Autodesk Inventor part; units mm, degrees
ref_plane "YZ Plane" through (0, 0, 0) normal (1, 0, 0) x (0, 1, 0)
ref_plane "XZ Plane" through (0, 0, 0) normal (0, 1, 0) x (-1, 0, 0)
ref_plane "XY Plane" through (0, 0, 0) normal (0, 0, 1) x (1, 0, 0)
sketch "Sketch1" plane through (0, 0, 0) normal (0, 0, 1) x (1, 0, 0)
  line L0 (0, 6.1628) -> (0, 4.6128)
  line L1 (0, 0) -> (0, -5.3285)
  line L2 (0, -7.6236) -> (0, 6.1628)
  line L3 (7.7918, 0) -> (42.6907, 0)
  line L4 (6.1094, -12.088) -> (6.1094, -4.669)
  line L5 (-6.1094, -10.2236) -> (-6.1094, -4.5067)
  line L6 (0, -7.6236) -> (0, -10.2236)
  line L7 (0, -7.6236) -> (0, -5.0236) construction
  arc A0 (-6.1094, 5.0092) -> (-6.87, -3.5101) centre (0, 0.1701) ccw
  arc A1 (6.1094, -4.669) -> (4.9829, 6.1628) centre (0, 0.1701) ccw
  circle A2 centre (27.3823, 0) radius 1.6
  circle A3 centre (27.3823, 0) radius 1.6
  arc A4 (15.7262, -19.2861) -> (15.9651, 19.4308) centre (0.0053, 0.1701) ccw
  arc A5 (14.9776, -18.1086) -> (14.9776, 18.1086) centre (0, 0) ccw construction
  line L8 (25.0186, 0.0157) -> (19.4598, 0.0157) construction
  line L9 (22.9824, -8.2534) -> (24.1975, 0.0157) construction
  line L10 (24.1975, 0.0157) -> (22.8643, 8.3172) construction
  line L11 (28.9823, 0) -> (30.9823, 0) construction
  line L12 (33.1204, -3.5101) -> (30.9986, 0.1649)
  line L13 (39.4857, -3.5101) -> (33.1204, -3.5101)
  line L14 (39.4857, 0.1649) -> (37.3639, -3.5101)
  circle A6 centre (35.2258, 0) radius 1.9
  line L15 (30.9986, 0.1649) -> (33.1239, 3.846)
  line L16 (33.1239, 3.846) -> (39.4857, 3.8504)
  line L17 (37.3639, 3.8489) -> (39.4857, 0.1649)
  line L18 (39.4857, 0.1784) -> (39.4857, 3.8504)
  line L19 (39.4857, 3.8504) -> (39.4857, -3.5101)
  line L20 (39.4857, 3.8504) -> (39.4857, 5.8504)
  line L21 (39.4857, 5.8504) -> (23.6696, 8.2698)
  arc A7 (15.7262, -19.2861) -> (15.9651, 19.4308) centre (0, 0.1701) ccw
  line L22 (39.4857, -3.5101) -> (39.4857, -5.5101)
  line L23 (39.4857, -5.5101) -> (23.6696, -7.9296)
  line L24 (23.6696, -7.9296) -> (23.6696, 8.2698)
  line L25 (0, 6.1628) -> (0, -10.2236)
  line L26 (0, -12.323) -> (0, -15.7561)
  line L27 (10.9155, -5.0236) -> (17.2808, -5.0236)
  line L28 (17.2808, -8.6986) -> (15.159, -12.3736)
  circle A8 centre (13.0373, -8.6986) radius 1.9
  line L29 (8.7937, -8.6986) -> (10.9155, -5.0236)
  line L30 (17.2808, -12.3736) -> (10.9155, -12.3736)
  line L31 (10.9155, -12.3736) -> (8.7937, -8.6986)
  line L32 (15.159, -5.0236) -> (17.2808, -8.6986)
  line L33 (10.9155, -12.3736) -> (10.9155, -14.3736)
  line L34 (-6.1094, -10.2236) -> (-6.1094, -14.3736)
  line L35 (0, -14.3736) -> (0, -10.2236)
  line L36 (0, -14.3736) -> (0, -19.3736)
  line L37 (-6.1094, -19.3736) -> (-6.1094, -14.3736)
  line L38 (0, -19.3736) -> (0, -25.3736)
  line L39 (0, -25.3736) -> (-6.1094, -25.3736)
  line L40 (-6.1094, -25.3736) -> (-6.1094, -19.3736)
  arc A9 (-4.8255, 6.1628) -> (-6.1094, -4.5067) centre (0, 0.1701) ccw
  line L41 (-5.029, 6.1628) -> (-4.9829, 6.1628)
  line L42 (-4.8255, 6.1628) -> (0, 6.1628)
  dimension "d2" = 3.8
  dimension "d3" = 2
  dimension "d4" = 2
  dimension "d5" = 16
  dimension "d6" = 2
  dimension "d7" = 16
  dimension "d9" = 3.8
  dimension "d10" = 2
  dimension "d17" = 5
  dimension "d50" = 6
  dimension "d64" = 7.7937
  dimension "d65" = 15.388
revolve "Revolution1" add sketch "Sketch1" angle 360 about axis through (0, -12.323, 0) along (0, -1, 0) contours L0 L2 L1 L6 L35 L26 L36 L38 L39 L40 L37 L34 L5 A9 L42
sketch "Sketch2" plane through (0, 0, 0) normal (1, 0, 0) x (0, 1, 0)
  line L0 (-4.669, 0) -> (-6.7907, -3.675) construction
  line L1 (-6.7907, 3.675) -> (-4.669, 0) construction
  line L2 (-15.156, 0) -> (-13.156, 0) construction
  line L3 (-11.0343, -3.675) -> (-6.7907, -3.675) construction
  line L4 (-4.5067, -6.1094) -> (-4.5067, 6.1094) construction
  line L5 (-4.5067, -6.1094) -> (-4.5067, 6.1094) construction
  line L6 (-48.8073, 0) -> (-58.5119, 0) construction
  line L7 (-8.9125, 0) -> (-6.3144, -1.5) construction
  line L8 (-17.8945, -2.9836) -> (-21.3586, -2.9836)
  line L9 (-21.3586, -2.9836) -> (-23.0907, 0.0164)
  line L10 (-23.0907, 0.0164) -> (-21.3586, 3.0164)
  line L11 (-21.3586, 3.0164) -> (-17.8945, 3.0164)
  line L12 (-17.8945, 3.0164) -> (-16.1625, 0.0164)
  line L13 (-16.1625, 0.0164) -> (-17.8945, -2.9836)
  line L14 (23.6533, 6.6124) -> (23.3606, 8.9041) construction
  line L15 (29.9823, 11.5805) -> (34.9823, 11.5805) construction
  line L16 (24.1789, 0) -> (22.8458, 8.3015) construction
  line L17 (25, 0) -> (19.4412, 0) construction
  line L18 (25.1551, -0.0164) -> (29.5051, -0.0164) construction
  line L19 (23.6533, -6.0645) -> (23.6533, 6.6124) construction
  arc A0 (14.9776, -18.1086) -> (14.9776, 18.1086) centre (0, 0) ccw construction
  arc A1 (18.0021, -17.3472) -> (18.0021, 17.3472) centre (0, 0) ccw construction
  arc A2 (18.0021, -17.3472) -> (18.0021, 17.3472) centre (0, 0) ccw construction
  line L20 (22.9638, -8.2692) -> (24.1789, 0) construction
  circle A3 centre (29.5051, -0.0164) radius 4.35 construction
  line L21 (43.4694, -5.828) -> (23.3606, -8.9041) construction
  line L22 (43.4694, 5.828) -> (23.3606, 8.9041) construction
  line L23 (37.4871, -3) -> (35.7551, 0) construction
  line L24 (35.7551, 0) -> (37.4871, 3) construction
  line L25 (43.4694, 5.828) -> (43.4694, -5.828) construction
  circle A4 centre (39.2192, 0) radius 1.9 construction
  line L26 (25, 0) -> (20.4835, 0) construction
  line L27 (23.6533, -6.0645) -> (23.3606, -8.9041) construction
  line L28 (43.4694, 0) -> (43.4694, 5.828) construction
  line L29 (43.4694, -5.828) -> (43.4694, 5.828) construction
  line L30 (29.5346, 0.0703) -> (29.5346, 0.0867) construction
  line L31 (37.4871, 3) -> (43.4694, 3.5234) construction
  line L32 (37.4871, -3) -> (43.4694, -3.5234) construction
  circle A5 centre (-17.0481, 18.2856) radius 1.75
  line L33 (-15.4481, 18.2856) -> (-13.4481, 18.2856) construction
  line L34 (-11.3263, 14.6106) -> (-13.4481, 18.2856) construction
  line L35 (-13.4481, 18.2856) -> (-11.3263, 21.9606) construction
  circle A6 centre (-9.2045, 18.2856) radius 1.9
  line L36 (-4.961, 18.2856) -> (-7.0828, 14.6106) construction
  line L37 (-7.0828, 21.9606) -> (-4.961, 18.2856) construction
  line L38 (-11.3263, 21.9606) -> (-7.0828, 21.9606) construction
  line L39 (-11.3263, 14.6106) -> (-7.0828, 14.6106) construction
  line L40 (-9.2045, 18.2856) -> (-6.6065, 16.7856)
  line L41 (-7.4725, 15.2856) -> (-10.9366, 15.2856)
  line L42 (-10.9366, 15.2856) -> (-12.6686, 18.2856)
  line L43 (-12.6686, 18.2856) -> (-10.9366, 21.2856)
  line L44 (-10.9366, 21.2856) -> (-7.4725, 21.2856)
  line L45 (-7.4725, 21.2856) -> (-5.7404, 18.2856)
  line L46 (-5.7404, 18.2856) -> (-7.4725, 15.2856)
  circle A7 centre (-19.6266, 0.0164) radius 1.9 construction
  circle A8 centre (-9.9125, 0) radius 4.35
  line L47 (-8.9125, 0) -> (-9.9125, 0)
  line L48 (-8.9125, 0) -> (-7.9125, 0) construction
  line L49 (-23.0907, 0.0164) -> (-25.0907, 0.0164)
  point P0 (23.6533, 8.0944)
  point P1 (23.6533, -8.0944)
  point P2 (39.2192, 3)
  point P3 (39.2192, 0)
  point P4 (43.4694, -3)
  point P5 (43.4694, 3)
  dimension "d37" = 3
  dimension "d42" = 3.8
  dimension "d43" = 2
  dimension "d44" = 3.5
  dimension "d45" = 7.35
  dimension "d46" = 3
  dimension "d47" = 1
  dimension "d48" = 180
  dimension "d49" = 2
extrude "Extrusion1" cut sketch "Sketch2" along normal blind 10 contours L8 L9 L10 L11 L12 L13 | A8
sketch "Sketch4" plane through (0, 0, 0) normal (1, 0, 0) x (0, 0, -1)
  line L0 (0, -15.156) -> (0, -13.156) construction
  line L1 (0, -4.669) -> (3.675, -6.7907) construction
  line L2 (-3.675, -6.7907) -> (0, -4.669) construction
  line L3 (3.675, -11.0343) -> (3.675, -6.7907) construction
  line L4 (6.1094, -4.669) -> (-6.1094, -4.669) construction
  line L5 (6.1094, -4.669) -> (-6.1094, -4.669) construction
  line L6 (0, -8.9125) -> (1.5, -6.3144) construction
  line L7 (2.9836, -17.8945) -> (2.9836, -21.3586)
  line L8 (2.9836, -21.3586) -> (-0.0164, -23.0907)
  line L9 (-0.0164, -23.0907) -> (-3.0164, -21.3586)
  line L10 (-3.0164, -21.3586) -> (-3.0164, -17.8945)
  line L11 (-3.0164, -17.8945) -> (-0.0164, -16.1625)
  line L12 (-0.0164, -16.1625) -> (2.9836, -17.8945)
  circle A0 centre (-0.0164, -19.6266) radius 1.9
  circle A1 centre (0, -9.9125) radius 4.35
  line L13 (0, -8.9125) -> (0, -9.9125)
  line L14 (0, -8.9125) -> (0, -7.9125) construction
  line L15 (-0.0164, -23.0907) -> (-0.0164, -25.0907)
  point P0 (0, -4.669)
  point P1 (6.1094, -4.669)
  point P2 (-6.1094, -4.669)
  point P3 (-0.0164, -23.0907)
  dimension "d51" = 3
  dimension "d52" = 1
  dimension "d53" = 180
  dimension "d54" = 2
extrude "Extrusion2" cut sketch "Sketch4" against normal blind 10 and the other way blind 5 contours A0 | A1
sketch "Sketch7" plane through (0, -25.3736, 0) normal (0, -1, 0) x (1, 0, 0)
  line L0 (0, 0.0164) -> (6.1094, 0.0164) construction
  line L1 (0, 0.0164) -> (-4, 0.0164) construction
  line L2 (-4, 0.0164) -> (-4, 4.0164) construction
  line L3 (-4, 4.0164) -> (0, 4.0164) construction
  line L4 (0, 4.0164) -> (0, 0.0164) construction
  line L5 (-4, 4.0164) -> (4, 4.0164)
  line L6 (4, 4.0164) -> (4, -3.9836)
  line L7 (4, -3.9836) -> (-4, -3.9836)
  line L8 (-4, -3.9836) -> (-4, 4.0164)
  line L9 (-4, -9.4779) -> (-8.9104, -9.4779)
  line L10 (-8.9104, -9.4779) -> (-8.9104, 10.8185)
  line L11 (-8.9104, 10.8185) -> (-4, 10.8185)
  line L12 (-4, 10.8185) -> (-4, -9.4779)
  line L13 (-7.8642, 4.0164) -> (7.4627, 4.0164)
  line L14 (7.4627, 4.0164) -> (7.4627, 9.8769)
  line L15 (7.4627, 9.8769) -> (-7.8642, 9.8769)
  line L16 (-7.8642, 9.8769) -> (-7.8642, 4.0164)
  line L17 (4, -8.5624) -> (10.7059, -8.5624)
  line L18 (10.7059, -8.5624) -> (10.7059, 4.0164)
  line L19 (10.7059, 4.0164) -> (4, 4.0164)
  line L20 (4, 4.0164) -> (4, -8.5624)
  line L21 (4, -12.198) -> (-4, -12.198)
  line L22 (-4, -12.198) -> (-4, -3.9836)
  line L23 (-4, -3.9836) -> (4, -3.9836)
  line L24 (4, -3.9836) -> (4, -12.198)
  dimension "d70" = 4
  dimension "d71" = 4
  dimension "d72" = 8
  dimension "d73" = 8
extrude "Extrusion5" cut sketch "Sketch7" against normal blind 10 contours L12 L15 L14 L13 L5 | L13 L16 L15 L12 | L8 L12 L9 L10 L11 L15 L16 L13 | L13 L19 L18 L17 L20 L6 | L7 L20 L24 L21 L22 L12
sketch "Sketch8" plane through (0, 6.1628, 0) normal (0, 1, 0) x (1, 0, 0)
  circle A0 centre (0, 0) radius 3.56
  dimension "d66" = 7.12
extrude "Extrusion6" cut sketch "Sketch8" against normal blind 10
properties part number "Now as three Part 2"
Can you work these out from the model? Positions are in its coordinate system, mm. A direction names the side the tool comes from. Round coordinates to 2 decimals unless told otherwise and drop trailing zeros. Write each loop counter-clockwise with the first axis right and the second up, starting at its lowest first coordinate (ties: lowest second). Pieces come first, ordered by that corner, then holes. Notation, with made-up numbers: (-18.75, -30) -> (29.25, -30) arc R22 ccw to (29.25, -4) -> close; hole circle Ø5 at (57.25, 61). An arc over 180 degrees is marked (long way). Use one line per item in the form item = value. Start each with the question number.
Q1. Imagine slicing it at A-A (y = -8.5). Please give me the cut outline in (x, z), then the cut area to 3 significant figures.
Q2. We'd pull the mould along Z, two halves only. Please class faces 6 (the face through (0, -18.1, 1.4)), 7 (the face through (0, -20, 4.016)), 8 (the face through (-4, -22, 0)): +Z half, -Z half, draft (parallel to the pull), parting line (faces both ways), or undercut.
Q3. If I drill on probe 1 along Y at (x, z) = (-3, 0); probe 2 along X at (y, z) = (-2.5, -1.5); probe 3 along Z at (x, y) = (-3.25, -10), over which ranges is the centre line in solid material (lowest first)? Write a range as [from, to].
Q4. I'm going to push flat-ended pins straight in: P1, Ø3, axis at x = -1, y = -7.5, coming from the +Z side; P2, Ø1, axis at x = -5.5, y = -3, coming from the +Z side; P3, Ø8, axis at x = -2.5, y = -11.5, coming from the -Z side. Where does each tip first touch, or does it pass through?
Q5. Imagine slicing it at B-B (z = -1). Count the separate pieces of the cut face and the enclosed holes in it, then the cut area to 3 significant figures.
Q6. Which directions (+Z, -Z, +X, -X, +Y, -Y) give clear straight access to the entire face, cutting with the end or side of a thin tool? Please do faces 1 (the face through (1.972, -22.237, 1.495)), 2 (the face through (0, -20, -3.984)), 3 (the face through (4, -23, 1)), 4 (the face through (0, -3.837, 0)), 5 (the face through (-1.97, -21.48, 0.43)).
Worked out:
q1.outline = (-4.52, -4.11) arc R6.11 ccw to (4.52, -4.11) -> close; (-4.52, 4.11) -> (4.52, 4.11) arc R6.11 ccw to start
q1.area = 24.9 mm^2
q2.face_6 = undercut
q2.face_7 = +Z half
q2.face_8 = draft
q3.probe_1 = [-25.37, -21.53], [-17.73, -14.26], [-5.56, -3.84]
q3.probe_2 = [-7.06, -3.23], [3.23, 7.06]
q3.probe_3 = [-5.17, -4.35], [4.35, 5.17]
q4.P1 = 6.11
q4.P2 = 5
q4.P3 = -6.11
q5.separate_pieces = 3
q5.enclosed_holes = 0
q5.area = 152 mm^2
q6.face_1 = +X
q6.face_2 = -Z, +X, -X, -Y
q6.face_3 = +Z, -Z, +X, -Y
q6.face_4 = +Y
q6.face_5 = +X, -X
